The listing builds one solid part. Answer for the finished solid, in the listing's coordinates (mm). Face numbers are marked on the shaded views. A direction names the side the tool comes from. Give positions to 0.01 mm unless a question says otherwise; leave off trailing zeros. Loops run counter-clockwise (first coordinate to the right, second up) from the corner with the lowest first, then second, coordinate; pieces in that order, holes last. Notation, with made-up numbers: M 59.25,25 L 83.25,25 A4 cw 83.25,29 Z; hole C -12.75,-18.75 d10. An arc over 180 degrees is marked long. One line per item, written item: value. Start each with the question number.
Q1. A cutting plane is placed at D-D, the plane z = 4. Determine the outline of the cut face in (x, y), and give its area (3 significant figures).
Q2. A cutting plane is placed at C-C, the plane z = -11.5. Determine the outline of the cut face in (x, y).
Q3. A cutting plane is placed at A-A, the plane x = 0. Determine the outline of the cut face in (y, z), and give its area (3 significant figures).
Q4. Consider L1, parallel to Y at x = 0, z = 5; L2, parallel to Y at x = 0, z = -15. Determine where each line is inside the solid, lowest interval first.
Q5. The mould has two halves that part along Y. Classify the marked faces 3, 4 and 5: +Y half, -Y half, draft (parallel to the pull), parting line (faces both ways), or undercut.
Q6. For the marked faces 1 and 2, determine the directions among +Z, -Z, +X, -X, +Y, -Y from which every point of the face is accessible in a straight line to the end or side of a thin tool.
Q7. Flat-ended cylindrical pins translate along their axes: pin 1 (8 mm diameter, centred on x = -9.5, z = -10.5, fed in from -Y); pin 2 (3 mm diameter, centred on x = 13.5, y = 3.5, fed in from -Z); pin 3 (6 mm diameter, centred on x = -11, y = -18, fed in from -Z); pin 4 (5 mm diameter, centred on x = 0, y = 0, fed in from -Z). Find the tip coordinate at first contact, or state that the pin passes through.
from build123d import *

# Parameters (mm, degrees)
F2_T = -2


# Not quite as in the source:
# - the program builds the solid bodies; features that only make, move or delete a surface that nothing else refers to are left out


with BuildPart() as f1:
    # F0 (on Right) → F1 (revolve)
    with BuildSketch(Plane.YZ):
        Polygon((0, 15.9718455747), (-5, 15.9718455747), (-5, 0.9718455747), (-26.5, -7.9165611044), (-26.5, -17.9165611044), (0, -17.9165611044), align=None)
    revolve(axis=Axis((0, 0, -0.4027476534), (0, 0, -1)))

    # F2
    f2_openings = [f1.faces().sort_by_distance(p)[0] for p in [
        (0, 0, -17.916561),
        (0, 0, 15.971846),
    ]]
    offset(amount=F2_T, openings=f2_openings, kind=Kind.INTERSECTION)


solid = f1.part
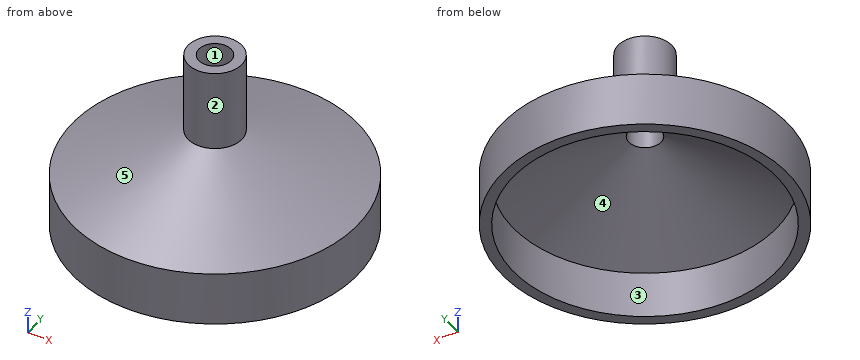
Answer block:
1. outline: C 0,0 d10; hole C 0,0 d6
1. area: 50.3 mm^2
2. outline: C 0,0 d53; hole C 0,0 d49
3. outline: M -26.5,-17.92 L -24.5,-17.92 L -24.5,-9.25 L -3,-0.37 L -3,15.97 L -5,15.97 L -5,0.97 L -26.5,-7.92 Z; M 3,-0.37 L 24.5,-9.25 L 24.5,-17.92 L 26.5,-17.92 L 26.5,-7.92 L 5,0.97 L 5,15.97 L 3,15.97 Z
3. area: 193 mm^2
4. L1: -5 to -3, 3 to 5
4. L2: -26.5 to -24.5, 24.5 to 26.5
5. face 3: undercut
5. face 4: undercut
5. face 5: parting line
6. face 1: +Z, -Z
6. face 2: +Z
7. pin 1: y = -25.92
7. pin 2: z = -5.51
7. pin 3: z = -9.09
7. pin 4: through
